Check sheet for the modelled part. Datum: model origin and axes. Units: mm. A direction names the side the tool comes from. Round coordinates to 2 decimals unless told otherwise and drop trailing zeros. Order: outer loops, then holes, each group sorted by start corner. A loop starts at its lowest first (then second) coordinate and runs counter-clockwise, first axis right, second up. Notation, with made-up numbers: (65, 67.5) -> (121, 67.5) arc R29 ccw to (121, 105.5) -> close; hole circle Ø11 at (-15.75, 20.25). An arc over 180 degrees is marked (long way). Answer in a Markdown table with one row per item.
from build123d import *

# Parameters (mm, degrees)
SKETCH1_W           = 7
SKETCH1_H           = 7
BOSS_EXTRUDE1_DEPTH = 3
CUT_EXTRUDE1_DEPTH  = 7
CUT_EXTRUDE2_DEPTH  = 11
SKETCH4_R           = 1.8
CUT_EXTRUDE3_DEPTH  = 0.8
CUT_EXTRUDE4_DEPTH  = 0.4


with BuildPart() as part:
    # Sketch1 → Boss-Extrude1 (new body)
    with BuildSketch(Plane(origin=(0, 0, 0), x_dir=(1, 0, 0), z_dir=(0, 1, 0))):
        with Locations((3.5, 3.5)):
            Rectangle(SKETCH1_W, SKETCH1_H)
    extrude(amount=BOSS_EXTRUDE1_DEPTH)

    # Sketch2 → Cut-Extrude1 (cut)
    with BuildSketch(Plane.XY):
        Polygon((0, 0), (0.7, 3), (0, 3), align=None)
        Polygon((7, 0), (6.3, 3), (7, 3), align=None)
    extrude(amount=-CUT_EXTRUDE1_DEPTH, mode=Mode.SUBTRACT)

    # Sketch3 → Cut-Extrude2 (cut)
    with BuildSketch(Plane(origin=(0, 0, 0), x_dir=(0, 0, -1), z_dir=(1, 0, 0))):
        Polygon((0, 0), (0.7, 3), (0, 3), align=None)
        Polygon((7, 3), (6.3, 3), (7, 0), align=None)
    extrude(amount=CUT_EXTRUDE2_DEPTH, mode=Mode.SUBTRACT)

    # Sketch4 → Cut-Extrude3 (cut)
    with BuildSketch(Plane.XZ):
        with Locations(Location((3.5, -3.5, 0), (0, 0, 270))):
            Circle(SKETCH4_R)
    extrude(amount=-CUT_EXTRUDE3_DEPTH, mode=Mode.SUBTRACT)

    # Sketch5 → Cut-Extrude4 (cut)
    with BuildSketch(Plane(origin=(0, 3, 0), x_dir=(1, 0, 0), z_dir=(0, 1, 0))):
        with BuildLine():
            Line((3.912067399, 5.252535384), (4.585144322, 5.252535384))
            Line((4.585144322, 5.252535384), (4.585144322, 3.046105095))
            add(Edge.make_bspline(
                [(4.585144322, 3.046105095), (4.584843541, 3.011045712), (4.584259872, 2.943012724), (4.580673506, 2.844127733), (4.575337598, 2.751510265), (4.567129137, 2.665173613), (4.555562948, 2.585304416), (4.543305201, 2.511265579), (4.528422816, 2.443431307), (4.515086598, 2.400993469), (4.508722046, 2.380740512)],
                knots=[0, 0, 0, 0, 1.251619961, 2.428777588, 3.532126049, 4.56323557, 5.523704531, 6.412540087, 7.242403515, 8, 8, 8, 8], degree=3))
            add(Edge.make_bspline(
                [(4.508722046, 2.380740512), (4.499827513, 2.355783352), (4.482224719, 2.306391691), (4.448010513, 2.235936597), (4.408665944, 2.169234852), (4.364301741, 2.105997397), (4.315336945, 2.04597069), (4.260110759, 1.990736894), (4.200565892, 1.938369412), (4.135027413, 1.891038204), (4.06514476, 1.846907146), (3.988927236, 1.810138919), (3.907874454, 1.778333915), (3.821306158, 1.752500626), (3.729197248, 1.73228764), (3.631783693, 1.717575234), (3.528935725, 1.70921534), (3.458690461, 1.708189441), (3.422684386, 1.707663589)],
                knots=[0, 0, 0, 0, 0.925533072, 1.831683394, 2.73255258, 3.630007683, 4.529542467, 5.436465751, 6.357118906, 7.298274949, 8.259461937, 9.242242071, 10.251058183, 11.300341426, 12.396409345, 13.544807631, 14.74152597, 16, 16, 16, 16], degree=3))
            add(Edge.make_bspline(
                [(3.422684386, 1.707663589), (3.380583904, 1.708681136), (3.298736769, 1.71065934), (3.179715358, 1.723792805), (3.068099561, 1.746763788), (2.964225235, 1.779943292), (2.867030957, 1.8211886), (2.777692308, 1.872636461), (2.695734484, 1.93325469), (2.62169044, 2.003229079), (2.555523571, 2.081852015), (2.498409733, 2.169813315), (2.449935297, 2.266193101), (2.410873173, 2.371427394), (2.380033539, 2.485012376), (2.357789346, 2.607187203), (2.344515975, 2.738021444), (2.342560592, 2.828024877), (2.341554578, 2.874330256)],
                knots=[0, 0, 0, 0, 1.114068574, 2.165849827, 3.164101702, 4.124467949, 5.046988974, 5.952942428, 6.846011651, 7.738523925, 8.642829306, 9.558838605, 10.50752403, 11.491963144, 12.524197802, 13.618364352, 14.774685164, 16, 16, 16, 16], degree=3))
            Line((2.341554578, 2.874330256), (3.014631501, 2.919202051))
            add(Edge.make_bspline(
                [(3.014631501, 2.919202051), (3.015840364, 2.894415849), (3.018158425, 2.846886919), (3.024594885, 2.778371834), (3.032733918, 2.715398444), (3.043383675, 2.658155757), (3.054852287, 2.60616009), (3.069750194, 2.560434701), (3.085412304, 2.519371749), (3.099168906, 2.495346649), (3.105777335, 2.483805416)],
                knots=[0, 0, 0, 0, 1.326609226, 2.543847584, 3.678365909, 4.719972403, 5.656527627, 6.521948534, 7.28997025, 8, 8, 8, 8], degree=3))
            add(Edge.make_bspline(
                [(3.105777335, 2.483805416), (3.115894166, 2.468540683), (3.135805351, 2.438497786), (3.17212863, 2.399348731), (3.211125287, 2.365122439), (3.254928677, 2.338213709), (3.302319529, 2.317050802), (3.353653599, 2.301673045), (3.408789357, 2.292348698), (3.446718972, 2.2914549), (3.466153937, 2.290996922)],
                knots=[0, 0, 0, 0, 1.023658308, 2.014687051, 2.979722519, 3.920049697, 4.880550909, 5.878122304, 6.912759386, 8, 8, 8, 8], degree=3))
            add(Edge.make_bspline(
                [(3.466153937, 2.290996922), (3.485804159, 2.291363098), (3.523578154, 2.292067004), (3.578014864, 2.298467893), (3.628066722, 2.308839798), (3.673760989, 2.323419076), (3.715252451, 2.342345121), (3.751621411, 2.366557721), (3.784435046, 2.393802377), (3.812780846, 2.426575807), (3.836932023, 2.466065164), (3.857097159, 2.514128918), (3.874444677, 2.57096477), (3.887851723, 2.637004807), (3.899263762, 2.7116168), (3.906422298, 2.795460452), (3.911567905, 2.88828796), (3.911896247, 2.953314858), (3.912067399, 2.987210865)],
                knots=[0, 0, 0, 0, 0.980314827, 1.884477813, 2.730827652, 3.527503874, 4.27366112, 4.998269146, 5.70163477, 6.396145331, 7.150281155, 8.001758491, 8.990432449, 10.111292654, 11.361572691, 12.75538406, 14.308707205, 16, 16, 16, 16], degree=3))
            Line((3.912067399, 2.987210865), (3.912067399, 5.252535384))
        make_face()
    extrude(amount=-CUT_EXTRUDE4_DEPTH, mode=Mode.SUBTRACT)


solid = part.part
Item 1: Cross-section at C-C (x = 4.75). Record the boundary of the cut face in (y, z), and give its area (3 significant figures).
Result sheet:
| item | result |
|---|---|
| outline | (0, -7) -> (3, -6.3) -> (3, -0.7) -> (0, 0) -> (0, -2.2) -> (0.8, -2.2) -> (0.8, -4.8) -> (0, -4.8) -> close |
| area | 16.8 mm^2 |
Item 2: Cross-section at B-B (z = -3.5). Record the boundary of the cut face in (x, y), and give its area (3 significant figures).
Result sheet:
| item | result |
|---|---|
| outline | (0, 0) -> (1.7, 0) -> (1.7, 0.8) -> (5.3, 0.8) -> (5.3, 0) -> (7, 0) -> (6.3, 3) -> (4.59, 3) -> (4.59, 2.6) -> (3.91, 2.6) -> (3.91, 3) -> (0.7, 3) -> close |
| area | 15.8 mm^2 |
Item 3: Cross-section at D-D (z = -4.5). Record the boundary of the cut face in (x, y).
Result sheet:
| item | result |
|---|---|
| outline | (0, 0) -> (2, 0) -> (2, 0.8) -> (5, 0.8) -> (5, 0) -> (7, 0) -> (6.3, 3) -> (4.59, 3) -> (4.59, 2.6) -> (3.91, 2.6) -> (3.91, 3) -> (0.7, 3) -> close |
Item 4: Depth check by flat-ended pin: P1, Ø1.1, axis at x = 3, z = -3, coming from the -Y side; P2, Ø1, axis at y = 2.5, z = -2.5, coming from the +X side. Enter the tip coordinate at first touch or a pass-through.
Result sheet:
| item | result |
|---|---|
| P1 | stops at y = 0.8 |
| P2 | stops at x = 6.53 |
Item 5: Set-up check for faces 5 (the cylindrical face through (4.041, 0.394, -5.217)), 6 (the flat face through (3, 3, -4)): record each of +Z, -Z, +X, -X, +Y, -Y from which the full face is reachable in a straight line by a thin tool's end or side.
Result sheet:
| item | result |
|---|---|
| face 5 | -Y |
| face 6 | +Z, -Z, +X, -X, +Y |
Item 6: Scan lines: line 1 (Y direction, x = 3.5, z = -1.75); line 2 (X direction, y = 0.4, z = -3.5); line 3 (Y direction, x = 3.75, z = -4.75). Record each from-to range of solid material in increasing order. Write a range as [from, to].
Result sheet:
| item | result |
|---|---|
| line 1 | y = [0.8, 2.6] |
| line 2 | x = [0.09, 1.7], [5.3, 6.91] |
| line 3 | y = [0.8, 3] |
Item 7: Mould release check, pull along Z, two halves, no side actions. Record for faces 1 (the flat face through (3.451, 1.521, -6.645)), 2 (the flat face through (4.2, 2.6, -3.1)), 3 (the flat face through (4, 0.8, -3)), 4 (the flat face through (6.655, 1.479, -3.451)): pulls with the +Z half, pulls with the -Z half, needs draft (parallel to the pull), parting line crosses it, or undercut.
Result sheet:
| item | result |
|---|---|
| face 1 | pulls with the -Z half |
| face 2 | undercut |
| face 3 | undercut |
| face 4 | needs draft |
Item 8: Cross-section at A-A (y = 0.4). Record the boundary of the cut face in (x, z), and give its area (3 significant figures).
Result sheet:
| item | result |
|---|---|
| outline | (0.09, -6.91) -> (6.91, -6.91) -> (6.91, -0.09) -> (0.09, -0.09) -> close; hole circle Ø3.6 at (3.5, -3.5) |
| area | 36.2 mm^2 |
